```python
from build123d import *

# Parameters (mm, degrees)
F2_R = 2.54
F3_T = -2


with BuildPart() as f1:
    # F0 (on Front) → F1 (revolve)
    with BuildSketch(Plane.XZ):
        Polygon((0, 150.7095229592), (0, 0.7095229592), (24, 0.7095229592), (24, 98.7095229592), (12, 110.7095229592), (12, 150.7095229592), align=None)
    revolve(axis=Axis((0, 0, 75.7095229592), (0, 0, -1)))

    # F2
    f2_edges = [f1.edges().sort_by_distance(p)[0] for p in [
        (-24, 0, 0.709523),
    ]]
    fillet(f2_edges, radius=F2_R)

    # F3
    f3_openings = [f1.faces().sort_by_distance(p)[0] for p in [
        (0, 0, 150.709523),
    ]]
    offset(amount=F3_T, openings=f3_openings, kind=Kind.INTERSECTION)


solid = f1.part
```
Work out the finished part from the listing and answer in its coordinate system (mm). A direction names the side the tool comes from. Give positions to 0.01 mm unless a question says otherwise; leave off trailing zeros. Write each loop counter-clockwise with the first axis right and the second up, starting at its lowest first coordinate (ties: lowest second). Pieces come first, ordered by that corner, then holes.
(1) Straight lines are drawn through the part: line 1 (Y direction, x = 0, z = 23); line 2 (Z direction, x = 2.5, y = -5.5). For each, find the intervals that lie inside material, in ascending order.
Final values:
line 1: y = -24 to -22, 22 to 24
line 2: z = 0.71 to 2.71
(2) The part is cut by section C-C on z = 18. Write down the section's boundary in (x, y), plus the area to 3 significant figures.
Final values:
outline: circle Ø48 at (0, 0); hole circle Ø44 at (0, 0)
area: 289 mm2
(3) The part is cut by section D-D on z = 103. Write down the section's boundary in (x, y).
Final values:
outline: circle Ø39.42 at (0, 0); hole circle Ø33.76 at (0, 0)
(4) Which of the six approach directions +Z, -Z, +X, -X, +Y, -Y give full straight-line access (tool end or side, diameter ignored) to faces 4 (the conical face through (-1.38, -10.49, 109.3)), 5 (the flat face through (0, 0, 0.71)), 6 (the cylindrical face through (-2.17, 9.76, 130.58))?
Final values:
face 4: none
face 5: -Z, +X, -X, +Y, -Y
face 6: +Z
(5) The part is cut by section A-A on y = 0. Write down the section's boundary in (x, z), plus the area to 3 significant figures.
Final values:
outline: (-24, 3.25) arc R2.54 ccw to (-21.46, 0.71) - (21.46, 0.71) arc R2.54 ccw to (24, 3.25) - (24, 98.71) - (12, 110.71) - (12, 150.71) - (10, 150.71) - (10, 109.88) - (22, 97.88) - (22, 3.25) arc R0.54 cw to (21.46, 2.71) - (-21.46, 2.71) arc R0.54 cw to (-22, 3.25) - (-22, 97.88) - (-10, 109.88) - (-10, 150.71) - (-12, 150.71) - (-12, 110.71) - (-24, 98.71) - close
area: 705 mm2
(6) The mould has two halves that part along X. Classify faces 1 (the flat face through (-5, -9, 150.71)), 2 (the conical face through (-2.73, 12.28, 110.13)), 3 (the flat face through (0, 0, 2.71)): pulls with the +X half, pulls with the -X half, needs draft (parallel to the pull), parting line crosses it, or undercut.
Final values:
face 1: needs draft
face 2: parting line crosses it
face 3: undercut
(7) Flat-ended cylindrical pins translate along their axes: pin 1 Ø12 at (y, z) = (-11.5, 26) entering from -X; pin 2 Ø4 at (y, z) = (1.5, 116.5) entering from -X; pin 3 Ø2 at (x, z) = (-3.5, 61.5) entering from +Y. Find the tip coordinate at first contact, or state that the pin passes through.
Final values:
pin 1: stops at x = -23.36
pin 2: stops at x = -12
pin 3: stops at y = 23.87
